Geometry check sheet. Reference: the model listing, model coordinates, mm. A direction names the side the tool comes from. Round coordinates to 2 decimals unless told otherwise and drop trailing zeros. Loops run counter-clockwise (first coordinate to the right, second up) from the corner with the lowest first, then second, coordinate; pieces in that order, holes last.
```python
from build123d import *

# Parameters (mm, degrees)
SKETCH1_R           = 4.4196
BOSS_EXTRUDE1_DEPTH = 7.9375
CUT_EXTRUDE1_DEPTH  = 201.660251187
FILLET1_R           = 12.7
SKETCH3_R           = 6.477
SKETCH3_R_2         = 2.20345
CUT_EXTRUDE2_DEPTH  = 201.660251187


with BuildPart() as part:
    # Sketch1 → Boss-Extrude1 (new body)
    with BuildSketch(Plane(origin=(0, 0, 0), x_dir=(1, 0, 0), z_dir=(0, 1, 0))):
        Polygon((-112.253201513, -112.253201513), (-58.371664787, -166.13473824), (58.371664787, -166.13473824), (112.253201513, -112.253201513), (112.253201513, 58.371664787), (0, -53.881536726), (-112.253201513, 58.371664787), align=None)
        with Locations(Location((-85.31243315, -112.253201513, 0), (0, 0, 270))):
            Circle(SKETCH1_R, mode=Mode.SUBTRACT)
        with Locations(Location((-58.371664787, -85.31243315, 0), (0, 0, 270))):
            Circle(SKETCH1_R, mode=Mode.SUBTRACT)
        with Locations(Location((-31.430896424, -112.253201513, 0), (0, 0, 270))):
            Circle(SKETCH1_R, mode=Mode.SUBTRACT)
        with Locations(Location((-58.371664787, -139.193969877, 0), (0, 0, 270))):
            Circle(SKETCH1_R, mode=Mode.SUBTRACT)
        with Locations(Location((31.430896424, -112.253201513, 0), (0, 0, 270))):
            Circle(SKETCH1_R, mode=Mode.SUBTRACT)
        with Locations(Location((58.371664787, -85.31243315, 0), (0, 0, 270))):
            Circle(SKETCH1_R, mode=Mode.SUBTRACT)
        with Locations(Location((85.31243315, -112.253201513, 0), (0, 0, 270))):
            Circle(SKETCH1_R, mode=Mode.SUBTRACT)
        with Locations(Location((58.371664787, -139.193969877, 0), (0, 0, 270))):
            Circle(SKETCH1_R, mode=Mode.SUBTRACT)
        with Locations(Location((-85.31243315, 4.490128061, 0), (0, 0, 270))):
            Circle(SKETCH1_R, mode=Mode.SUBTRACT)
        with Locations(Location((-58.371664787, -22.450640303, 0), (0, 0, 270))):
            Circle(SKETCH1_R, mode=Mode.SUBTRACT)
        with Locations(Location((58.371664787, -22.450640303, 0), (0, 0, 270))):
            Circle(SKETCH1_R, mode=Mode.SUBTRACT)
        with Locations(Location((85.31243315, 4.490128061, 0), (0, 0, 270))):
            Circle(SKETCH1_R, mode=Mode.SUBTRACT)
    extrude(amount=BOSS_EXTRUDE1_DEPTH)

    # Sketch2 → Cut-Extrude1 (cut, through all)
    with BuildSketch(Plane(origin=(0, 7.9375, 0), x_dir=(1, 0, 0), z_dir=(0, 1, 0))):
        Polygon((0, -53.881536726), (-112.253201513, 58.371664787), (-112.253201513, 51.18745989), (0, -61.065741623), (112.253201513, 51.18745989), (112.253201513, 58.371664787), align=None)
    extrude(amount=-CUT_EXTRUDE1_DEPTH, mode=Mode.SUBTRACT)

    # Fillet1
    fillet1_edges = [part.edges().sort_by_distance(p)[0] for p in [
        (112.253201513, 3.96875, 112.253201513),
        (58.371664787, 3.96875, 166.13473824),
        (-58.371664787, 3.96875, 166.13473824),
        (-112.253201513, 3.96875, 112.253201513),
        (0, 3.96875, 61.065741623),
        (-112.253201513, 3.96875, -51.18745989),
        (112.253201513, 3.96875, -51.18745989),
    ]]
    fillet(fillet1_edges, radius=FILLET1_R)

    # Sketch3 → Cut-Extrude2 (cut, through all)
    with BuildSketch(Plane(origin=(0, 7.9375, 0), x_dir=(1, 0, 0), z_dir=(0, 1, 0))):
        with Locations(Location((0, -133.99727835, 0), (0, 0, 270))):
            Circle(SKETCH3_R)
        with Locations(Location((-10.31875, -133.99727835, 0), (0, 0, 270))):
            Circle(SKETCH3_R_2)
        with Locations(Location((10.31875, -133.99727835, 0), (0, 0, 270))):
            Circle(SKETCH3_R_2)
        with Locations(Location((-76.332177029, -57.665101321, 0), (0, 0, 270))):
            Circle(SKETCH3_R)
        with Locations(Location((-69.035718931, -64.961559419, 0), (0, 0, 270))):
            Circle(SKETCH3_R_2)
        with Locations(Location((-83.628635127, -50.368643222, 0), (0, 0, 270))):
            Circle(SKETCH3_R_2)
        with Locations(Location((76.332177029, -57.665101321, 0), (0, 0, 270))):
            Circle(SKETCH3_R)
        with Locations(Location((69.035718931, -64.961559419, 0), (0, 0, 270))):
            Circle(SKETCH3_R_2)
        with Locations(Location((83.628635127, -50.368643222, 0), (0, 0, 270))):
            Circle(SKETCH3_R_2)
    extrude(amount=-CUT_EXTRUDE2_DEPTH, mode=Mode.SUBTRACT)


solid = part.part
```
1) Sectioned sample at A-A, the plane x = 0. Record the cut outline in (y, z).
Report:
outline: (0, 55.81) - (7.94, 55.81) - (7.94, 127.52) - (0, 127.52) - close; (0, 140.47) - (7.94, 140.47) - (7.94, 166.13) - (0, 166.13) - close
2) Access from +Z, -Z, +X, -X, +Y, -Y to the whole of each face (thin tool, end or side, straight path). Record for faces 1 (the face through (49.205, 4.024, 11.86)), 2 (the face through (57.907, 4.024, 165.195)).
Report:
face 1: -Z, +Y, -Y
face 2: +Z, +X, +Y, -Y
3) Scan lines: line 1 along X through (y, z) = (2.25, 114); line 2 along X through (y, z) = (4.75, 141); line 3 along X through (y, z) = (2.5, 130). Record each from-to range of solid material in increasing order.
Report:
line 1: x = -110.15 to -89.37, -81.25 to -35.49, -27.37 to 27.37, 35.49 to 81.25, 89.37 to 110.15
line 2: x = -83.51 to -62.41, -54.34 to 54.34, 62.41 to 83.51
line 3: x = -94.51 to -5.1, 5.1 to 94.51
4) Gauge pin test, flat ends, axial feed: pin 1 (2 mm diameter, centred on x = -28, y = 6.5, fed in from -Z); pin 2 (2 mm diameter, centred on x = -29.5, y = 7, fed in from -Z); pin 3 (1 mm diameter, centred on y = 3, z = 136.5, fed in from +X). Record the tip position at first contact, or that the pin passes through.
Report:
pin 1: stops at z = 32.07
pin 2: stops at z = 30.57
pin 3: stops at x = 88.51
5) Sectioned sample at B-B, the plane y = 3.25. State how many separate pieces and enclosed holes the cut face has, then the cut area to 3 significant figures.
Report:
separate pieces: 1
enclosed holes: 21
area: 31,700 mm2
6) Mould release check, pull along Z, two halves, no side actions. Record for faces 3 (the face through (-0.14, 3.913, 55.804)), 4 (the face through (31.63, 3.91, 107.84)), 5 (the face through (84.987, 3.913, 139.519)): +Z half, -Z half, draft (parallel to the pull), parting line (faces both ways), or undercut.
Report:
face 3: -Z half
face 4: undercut
face 5: +Z half
